Geometry check sheet. Reference: drawing and pictorial views, mm from the part's lowest x, y, z. A direction names the side the tool comes from. Round coordinates to 2 decimals unless told otherwise and drop trailing zeros. Write each loop counter-clockwise with the first axis right and the second up, starting at its lowest first coordinate (ties: lowest second). Pieces come first, ordered by that corner, then holes.
Item 1: Section check A-A, the plane z = 13.25. Record the cut outline in (x, y).
Item 2: Depth check by flat-ended pin: pin 1 (1.5 mm diameter, centred on x = 90, y = 41, fed in from +Z) (3 decimals); pin 2 (6 mm diameter, centred on y = 25.5, z = 19.5, fed in from +X); pin 3 (8 mm diameter, centred on y = 16.5, z = 6, fed in from -X). Enter the tip coordinate at first touch or a pass-through.
Item 3: Set-up check for the marked faces 4 and 5: record each of +Z, -Z, +X, -X, +Y, -Y from which the full face is reachable in a straight line by a thin tool's end or side.
Item 4: Section check D-D, the plane x = 85. Record the cut outline in (y, z) (1 decimal).
Item 5: Material ranges on line 1 along Z through (x, y) = (132.5, 39) (1 decimal); line 2 along X through (y, z) = (45, 4.25) (1 decimal); line 3 along Y through (x, z) = (110, 3) (1 decimal), recorded low to high.
Item 6: Release check for a two-part mould opening along X. For the marked faces 1, 2 and 3 record: pulls with the +X half, pulls with the -X half, needs draft (parallel to the pull), parting line crosses it, or undercut.
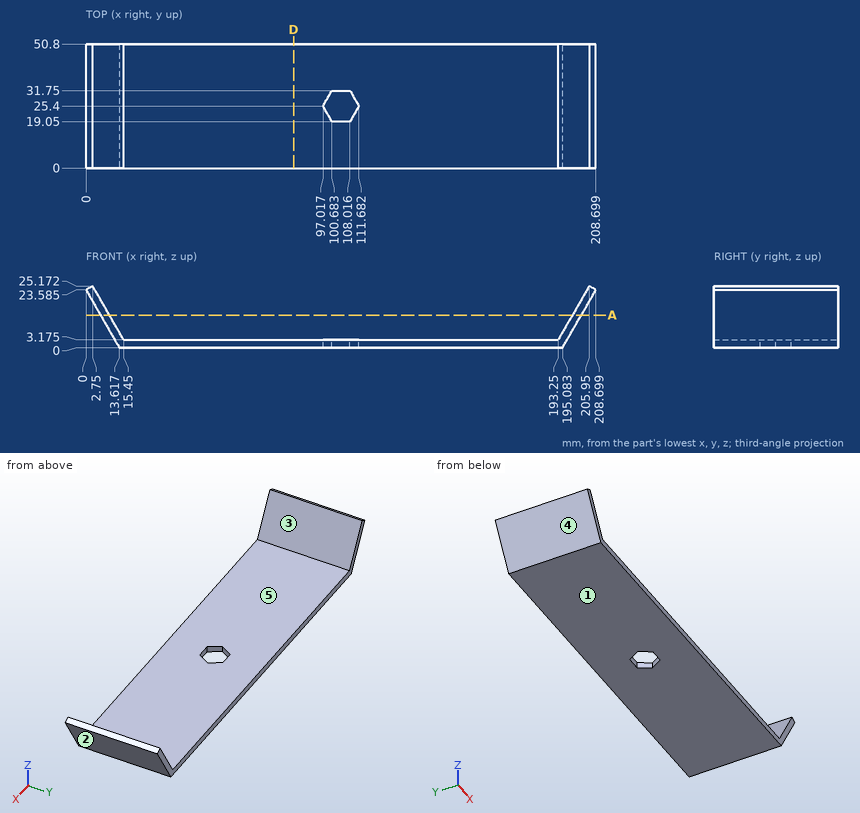
Values found:
1. outline: (5.97, 0) - (9.63, 0) - (9.63, 50.8) - (5.97, 50.8) - close; (199.07, 0) - (202.73, 0) - (202.73, 50.8) - (199.07, 50.8) - close
2. pin 1: stops at z = 3.175
2. pin 2: stops at x = 208.07
2. pin 3: stops at x = 7.84
3. face 4: -Z, -X, +Y, -Y
3. face 5: +Z, +Y, -Y
4. outline: (0, 0) - (50.8, 0) - (50.8, 3.2) - (0, 3.2) - close
5. line 1: z = 0 to 3.2
5. line 2: x = 11.2 to 14.8, 193.9 to 197.5
5. line 3: y = 0 to 22.5, 28.3 to 50.8
6. face 1: needs draft
6. face 2: pulls with the +X half
6. face 3: undercut
